Part model, mm, in its own coordinate system. Round coordinates to 2 decimals unless told otherwise and drop trailing zeros. Write each loop counter-clockwise with the first axis right and the second up, starting at its lowest first coordinate (ties: lowest second). Pieces come first, ordered by that corner, then holes.
```python
from build123d import *

# Parameters (mm, degrees)
AUFSATZ_LINEAR_AUSTRAGEN1_DEPTH = 5
SKIZZE11_R                      = 4.5
SCHNITT_LINEAR_AUSTRAGEN1_DEPTH = 3.5
SKIZZE12_R                      = 3
SCHNITT_LINEAR_AUSTRAGEN2_DEPTH = 1.5
SKIZZE13_W                      = 2.085762608
SKIZZE13_H                      = 3.10677117
AUFSATZ_LINEAR_AUSTRAGEN2_DEPTH = 6
SKIZZE14_W                      = 6
SKIZZE14_H                      = 3.10677117
AUFSATZ_LINEAR_AUSTRAGEN3_DEPTH = 1
SCHNITT_LINEAR_AUSTRAGEN3_DEPTH = 5
SKIZZE17_R                      = 1.5
AUFSATZ_LINEAR_AUSTRAGEN4_DEPTH = 10


with BuildPart() as part:
    # Skizze1 → Aufsatz-Linear austragen1 (new body)
    with BuildSketch(Plane(origin=(0, 0, 0), x_dir=(1, 0, 0), z_dir=(0, 1, 0))):
        with BuildLine():
            Line((0, 0), (0, -75))
            ThreePointArc((0, -75), (-37.5, -37.5), (0, 0))
        make_face()
    extrude(amount=AUFSATZ_LINEAR_AUSTRAGEN1_DEPTH)

    # Skizze11 → Schnitt-Linear austragen1 (cut)
    with BuildSketch(Plane(origin=(0, 5, 0), x_dir=(1, 0, 0), z_dir=(0, 1, 0))):
        with Locations((-18.75, -11.5)):
            Circle(SKIZZE11_R)
        with Locations((-18.75, -63.5)):
            Circle(SKIZZE11_R)
    extrude(amount=-SCHNITT_LINEAR_AUSTRAGEN1_DEPTH, mode=Mode.SUBTRACT)

    # Skizze12 → Schnitt-Linear austragen2 (cut)
    with BuildSketch(Plane(origin=(0, 1.5, 0), x_dir=(1, 0, 0), z_dir=(0, 1, 0))):
        with Locations((-18.75, -63.5)):
            Circle(SKIZZE12_R)
        with Locations((-18.75, -11.5)):
            Circle(SKIZZE12_R)
    extrude(amount=-SCHNITT_LINEAR_AUSTRAGEN2_DEPTH, mode=Mode.SUBTRACT)

    # Skizze13 → Aufsatz-Linear austragen2 (add)
    with BuildSketch(Plane(origin=(0, 5, 0), x_dir=(1, 0, 0), z_dir=(0, 1, 0))):
        with Locations((-12.416205268, -9.745021236)):
            Rectangle(SKIZZE13_W, SKIZZE13_H)
    extrude(amount=AUFSATZ_LINEAR_AUSTRAGEN2_DEPTH)

    # Skizze14 → Aufsatz-Linear austragen3 (add)
    with BuildSketch(Plane(origin=(0, 11, 0), x_dir=(1, 0, 0), z_dir=(0, 1, 0))):
        with Locations((-14.373323964, -9.745021236)):
            Rectangle(SKIZZE14_W, SKIZZE14_H)
    extrude(amount=AUFSATZ_LINEAR_AUSTRAGEN3_DEPTH)

    # Skizze16 → Schnitt-Linear austragen3 (cut)
    with BuildSketch(Plane(origin=(0, 12, 0), x_dir=(1, 0, 0), z_dir=(0, 1, 0))):
        with BuildLine():
            Line((-17.373323964, -11.298406821), (-13.43004884, -11.298406821))
            ThreePointArc((-13.43004884, -11.298406821), (-15.401686402, -9.326769259), (-17.373323964, -11.298406821))
        make_face()
    extrude(amount=-SCHNITT_LINEAR_AUSTRAGEN3_DEPTH, mode=Mode.SUBTRACT)

    # Skizze17 → Aufsatz-Linear austragen4 (add)
    with BuildSketch(Plane(origin=(0, 5, 0), x_dir=(1, 0, 0), z_dir=(0, 1, 0))):
        with Locations((-5.905120945, -20.937212942)):
            Circle(SKIZZE17_R)
    extrude(amount=AUFSATZ_LINEAR_AUSTRAGEN4_DEPTH)


solid = part.part
```
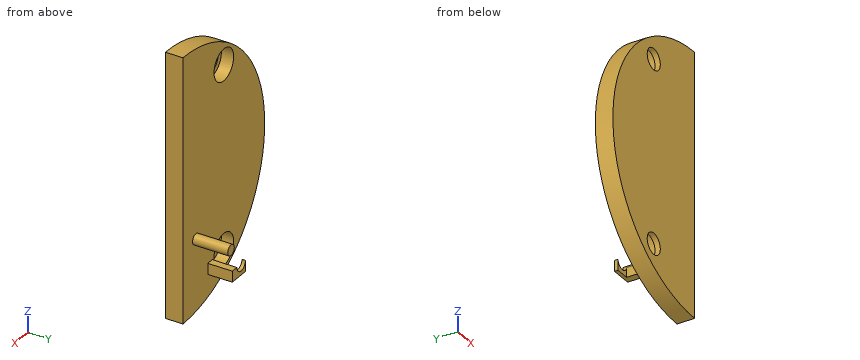
Q1. Cut at B-B on z = 63.5. Write the cut outline in (x, y), plus the area to 3 significant figures.
Values follow:
outline: (-27.02, 0) - (-21.75, 0) - (-21.75, 1.5) - (-23.25, 1.5) - (-23.25, 5) - (-27.02, 5) - close; (-15.75, 0) - (0, 0) - (0, 5) - (-14.25, 5) - (-14.25, 1.5) - (-15.75, 1.5) - close
area: 94.6 mm2
Q2. Cut at C-C on z = 37.5. Write the cut outline in (x, y).
Values follow:
outline: (-37.5, 0) - (0, 0) - (0, 5) - (-37.5, 5) - close
Q3. Cut at D-D on x = -26.5. Write the cut outline in (y, z).
Values follow:
outline: (0, 10.97) - (5, 10.97) - (5, 64.03) - (0, 64.03) - close
Q4. Drop flat-ended pins along their axis: pin 1 (5.5 mm diameter, centred on x = -18.75, z = 63.5, fed in from +Y); pin 2 (4.5 mm diameter, centred on x = -18.5, z = 12, fed in from +Y); pin 3 (1.6 mm diameter, centred on y = 9.5, z = 9.5, fed in from -X); pin 4 (8 mm diameter, centred on x = -9.5, y = 12.5, fed in from +Z). Give the stop position or say it passes through.
Values follow:
pin 1: passes through
pin 2: stops at y = 12
pin 3: stops at x = -13.46
pin 4: stops at z = 22.44
Q5. Cut at A-A on x = -20. Write the cut outline in (y, z), plus the area to 3 significant figures.
Values follow:
outline: (0, 5.78) - (5, 5.78) - (5, 7.18) - (1.5, 7.18) - (1.5, 8.77) - (0, 8.77) - close; (0, 14.23) - (1.5, 14.23) - (1.5, 15.82) - (5, 15.82) - (5, 59.18) - (1.5, 59.18) - (1.5, 60.77) - (0, 60.77) - close; (0, 66.23) - (1.5, 66.23) - (1.5, 67.82) - (5, 67.82) - (5, 69.22) - (0, 69.22) - close
area: 240 mm2
Q6. Wall check: L1, parallel to Z at x = -18.75, y = 2.8; L2, parallel to Z at x = -18.75, y = 0.95; L3, parallel to Y at x = -13.5, z = 35.5. Give the ranges that are in metal, low to high.
Values follow:
L1: z = 5.02 to 7, 16 to 59, 68 to 69.98
L2: z = 5.02 to 8.5, 14.5 to 60.5, 66.5 to 69.98
L3: y = 0 to 5
